Work out the finished part from the listing and answer in its coordinate system (mm). A direction names the side the tool comes from. Give positions to 0.01 mm unless a question says otherwise; leave off trailing zeros. Loops run counter-clockwise (first coordinate to the right, second up) from the corner with the lowest first, then second, coordinate; pieces in that order, holes last. Notation, with made-up numbers: (-15.5, 53) - (10.5, 53) arc R24 cw to (10.5, 68) - close; hole circle Ø3 at (-37, 37.5). An arc over 180 degrees is marked (long way). Use CSV: the item, a comma, the result in double quotes.
from build123d import *

# Parameters (mm, degrees)
SKETCH1_W           = 175
SKETCH1_H           = 43
BOSS_EXTRUDE1_DEPTH = 4
BOSS_EXTRUDE2_DEPTH = 43
SKETCH2_R           = 1.55
SKETCH2_W           = 24.921803412
SKETCH2_H           = 2.5
CUT_EXTRUDE1_DEPTH  = 43
SKETCH3_R           = 1.6
SKETCH3_R_2         = 8
SKETCH3_R_3         = 4.1
CUT_EXTRUDE2_DEPTH  = 43
SKETCH4_R           = 5
CUT_EXTRUDE3_DEPTH  = 43
CUT_EXTRUDE4_DEPTH  = 5
SKETCH6_W           = 101
SKETCH6_H           = 32.974785191
BOSS_EXTRUDE3_DEPTH = 3
CUT_EXTRUDE6_DEPTH  = 1.25
CUT_EXTRUDE7_DEPTH  = 3
CUT_EXTRUDE8_DEPTH  = 4
SKETCH4_4_R         = 4.1
CUT_EXTRUDE9_DEPTH  = 150
BOSS_EXTRUDE4_DEPTH = 60
CUT_EXTRUDE10_DEPTH = 50
BOSS_EXTRUDE5_DEPTH = 1.5
BOSS_EXTRUDE6_DEPTH = 3


with BuildPart() as part:
    # Sketch1 → Boss-Extrude1 (new body)
    with BuildSketch(Plane(origin=(0, 0, 0), x_dir=(1, 0, 0), z_dir=(0, 1, 0))):
        Rectangle(SKETCH1_W, SKETCH1_H)
        Polygon((77.5, -17.02423389), (-18.39852542, -17.02423389), (77.5, 12.216270532), align=None, mode=Mode.SUBTRACT)
        Polygon((-23.5, -13.411203118), (-23.5, 17.839340837), (77.209154002, 17.839340837), align=None, mode=Mode.SUBTRACT)
        Polygon((-33.5, -8.231428571), (-79.616903449, 16.459632181), (-33.5, 16.459632181), align=None, mode=Mode.SUBTRACT)
        Polygon((-80.5, -17.02423389), (-80.5, 9.251394926), (-36.98536512, -17.02423389), align=None, mode=Mode.SUBTRACT)
    extrude(amount=BOSS_EXTRUDE1_DEPTH)

    # Sketch1_3 → Boss-Extrude2 (add)
    with BuildSketch(Plane(origin=(0, 0, 0), x_dir=(1, 0, 0), z_dir=(0, 1, 0))):
        Polygon((-87.5, 21.5), (-87.5, -21.5), (-80.5, -21.5), (-80.5, -17.02423389), (-80.5, 9.251394926), (-80.5, 21.5), align=None)
        Polygon((-33.5, -8.231428571), (-33.5, -21.5), (-23.5, -21.5), (-23.5, -13.411203118), (-23.5, 17.839340837), (-23.5, 21.5), (-33.5, 21.5), (-33.5, 16.459632181), align=None)
        Polygon((77.5, -17.02423389), (77.5, -21.5), (87.5, -21.5), (87.5, 21.5), (77.5, 21.5), (77.5, 12.216270532), align=None)
    extrude(amount=-BOSS_EXTRUDE2_DEPTH)

    # Sketch2 → Cut-Extrude1 (cut)
    with BuildSketch(Plane(origin=(-80.5, 0, 0), x_dir=(0, 0, -1), z_dir=(1, 0, 0))):
        Polygon((21.5, -43), (21.5, -30.260907637), (14.145081595, -43), align=None)
        Polygon((-21.5, -43), (-14.145081595, -43), (-21.5, -30.260907637), align=None)
        with Locations((0, -34)):
            Circle(SKETCH2_R)
        with Locations((-10.825317547, -27.75)):
            Circle(SKETCH2_R)
        with Locations((-10.825317547, -15.25)):
            Circle(SKETCH2_R)
        with Locations((0, 2.75)):
            Rectangle(SKETCH2_W, SKETCH2_H)
        with Locations((0, -9)):
            Circle(SKETCH2_R)
        with Locations((10.825317547, -15.25)):
            Circle(SKETCH2_R)
        with Locations((10.825317547, -27.75)):
            Circle(SKETCH2_R)
    extrude(amount=-CUT_EXTRUDE1_DEPTH, mode=Mode.SUBTRACT)

    # Sketch3 → Cut-Extrude2 (cut)
    with BuildSketch(Plane(origin=(-23.5, 0, 0), x_dir=(0, 0, -1), z_dir=(1, 0, 0))):
        with Locations((15.5, -37)):
            Circle(SKETCH3_R)
        with Locations((0, -21.5)):
            Circle(SKETCH3_R_2)
        with BuildLine():
            Line((-8, -43), (8, -43))
            Line((8, -43), (8, -21.5))
            ThreePointArc((8, -21.5), (0, -29.5), (-8, -21.5))
            Line((-8, -21.5), (-8, -43))
        make_face()
        with Locations((18.5, -21.5)):
            Circle(SKETCH3_R_3)
        with Locations((15.5, -6)):
            Circle(SKETCH3_R)
        with Locations((-15.5, -6)):
            Circle(SKETCH3_R)
        with Locations((-18.5, -21.5)):
            Circle(SKETCH3_R_3)
        with Locations((-15.5, -37)):
            Circle(SKETCH3_R)
    extrude(amount=-CUT_EXTRUDE2_DEPTH, mode=Mode.SUBTRACT)

    # Sketch4 → Cut-Extrude3 (cut)
    with BuildSketch(Plane(origin=(87.5, 0, 0), x_dir=(0, 0, -1), z_dir=(1, 0, 0))):
        with Locations((0, -21.5)):
            Circle(SKETCH4_R)
        with BuildLine():
            ThreePointArc((21.5, -18.705362278), (16.998334258, -17.684898429), (14.4, -21.5))
            ThreePointArc((14.4, -21.5), (16.998334258, -25.315101571), (21.5, -24.294637722))
            Line((21.5, -24.294637722), (21.5, -18.705362278))
        make_face()
        with BuildLine():
            ThreePointArc((-21.5, -24.294637722), (-16.998334258, -25.315101571), (-14.4, -21.5))
            ThreePointArc((-14.4, -21.5), (-16.998334258, -17.684898429), (-21.5, -18.705362278))
            Line((-21.5, -18.705362278), (-21.5, -24.294637722))
        make_face()
        with BuildLine():
            Line((-6, -43), (6, -43))
            Line((6, -43), (6, -37.5))
            ThreePointArc((6, -37.5), (0, -31.5), (-6, -37.5))
            Line((-6, -37.5), (-6, -43))
        make_face()
    extrude(amount=-CUT_EXTRUDE3_DEPTH, mode=Mode.SUBTRACT)

    # Sketch4_3 → Cut-Extrude4 (cut)
    with BuildSketch(Plane(origin=(87.5, 0, 0), x_dir=(0, 0, -1), z_dir=(1, 0, 0))):
        with BuildLine():
            ThreePointArc((-8.05, -21.5), (0, -29.55), (8.05, -21.5))
            Line((8.05, -21.5), (5, -21.5))
            ThreePointArc((5, -21.5), (0, -26.5), (-5, -21.5))
            Line((-5, -21.5), (-8.05, -21.5))
        make_face()
        with BuildLine():
            Line((5, -21.5), (8.05, -21.5))
            ThreePointArc((8.05, -21.5), (0, -13.45), (-8.05, -21.5))
            Line((-8.05, -21.5), (-5, -21.5))
            ThreePointArc((-5, -21.5), (0, -16.5), (5, -21.5))
        make_face()
    extrude(amount=-CUT_EXTRUDE4_DEPTH, mode=Mode.SUBTRACT)

    # Sketch6 → Boss-Extrude3 (add)
    with BuildSketch(Plane(origin=(0, 0, -21.5), x_dir=(-1, 0, 0), z_dir=(0, 0, -1))):
        Polygon((87.5, -30.260907637), (80.5, -30.260907637), (33.5, -43), (23.5, -43), (-77.5, -43), (-87.5, -43), (-87.5, 4), (87.5, 4), align=None)
        with Locations((-27, -18.169210683)):
            Rectangle(SKETCH6_W, SKETCH6_H, mode=Mode.SUBTRACT)
        Polygon((80.5, -23.601473433), (80.5, -1.681818087), (33.5, -1.681818087), (33.5, -34.656603278), align=None, mode=Mode.SUBTRACT)
    boss_extrude3 = extrude(amount=BOSS_EXTRUDE3_DEPTH)

    # Mirror1: Boss-Extrude3 across plane
    add(boss_extrude3.mirror(Plane.XY))

    # Sketch7 → Cut-Extrude6 (cut, symmetric)
    with BuildSketch(Plane(origin=(81.5, 0, 0), x_dir=(0, 0, -1), z_dir=(1, 0, 0))):
        with BuildLine():
            Line((11.709666808, -33.5), (1.443160895, -31.162233309))
            ThreePointArc((1.443160895, -31.162233309), (0, -31), (-1.443160895, -31.162233309))
            Line((-1.443160895, -31.162233309), (-11.709666808, -33.5))
            ThreePointArc((-11.709666808, -33.5), (-12.278204733, -33.856933451), (-12.5, -34.490529316))
            Line((-12.5, -34.490529316), (-12.5, -59.657999149))
            Line((-12.5, -59.657999149), (12.5, -59.657999149))
            Line((12.5, -59.657999149), (12.5, -34.490529316))
            ThreePointArc((12.5, -34.490529316), (12.278204733, -33.856933451), (11.709666808, -33.5))
        make_face()
    extrude(amount=CUT_EXTRUDE6_DEPTH, both=True, mode=Mode.SUBTRACT)

    # Sketch8 → Cut-Extrude7 (cut)
    with BuildSketch(Plane.ZY.offset(33.5)):
        with BuildLine():
            Line((-8, -43), (-8, -21.5))
            ThreePointArc((-8, -21.5), (0, -13.5), (8, -21.5))
            Line((8, -21.5), (8, -43))
            Line((8, -43), (11.5, -43))
            Line((11.5, -43), (11.5, -21.5))
            ThreePointArc((11.5, -21.5), (0, -10), (-11.5, -21.5))
            Line((-11.5, -21.5), (-11.5, -43))
            Line((-11.5, -43), (-8, -43))
        make_face()
    extrude(amount=-CUT_EXTRUDE7_DEPTH, mode=Mode.SUBTRACT)

    # Sketch9 → Cut-Extrude8 (cut)
    with BuildSketch(Plane(origin=(-80.5, 0, 0), x_dir=(0, 0, -1), z_dir=(1, 0, 0))):
        Polygon((-2.9, -32.325684219), (-2.9, -35.674315781), (0, -37.348631561), (2.9, -35.674315781), (2.9, -32.325684219), (0, -30.651368439), align=None)
        Polygon((-10.825317547, -24.401368439), (-13.725317547, -26.075684219), (-13.725317547, -29.424315781), (-10.825317547, -31.098631561), (-7.925317547, -29.424315781), (-7.925317547, -26.075684219), align=None)
        Polygon((-10.825317547, -18.598631561), (-7.925317547, -16.924315781), (-7.925317547, -13.575684219), (-10.825317547, -11.901368439), (-13.725317547, -13.575684219), (-13.725317547, -16.924315781), align=None)
        Polygon((-2.9, -7.325684219), (-2.9, -10.674315781), (0, -12.348631561), (2.9, -10.674315781), (2.9, -7.325684219), (0, -5.651368439), align=None)
        Polygon((7.925317547, -13.575684219), (7.925317547, -16.924315781), (10.825317547, -18.598631561), (13.725317547, -16.924315781), (13.725317547, -13.575684219), (10.825317547, -11.901368439), align=None)
        Polygon((7.925317547, -26.075684219), (7.925317547, -29.424315781), (10.825317547, -31.098631561), (13.725317547, -29.424315781), (13.725317547, -26.075684219), (10.825317547, -24.401368439), align=None)
    extrude(amount=-CUT_EXTRUDE8_DEPTH, mode=Mode.SUBTRACT)

    # Sketch4_4 → Cut-Extrude9 (cut)
    with BuildSketch(Plane(origin=(87.5, 0, 0), x_dir=(0, 0, -1), z_dir=(1, 0, 0))):
        with Locations((18.5, -21.5)):
            Circle(SKETCH4_4_R)
        with Locations((-18.5, -21.5)):
            Circle(SKETCH4_4_R)
    extrude(amount=-CUT_EXTRUDE9_DEPTH, mode=Mode.SUBTRACT)

    # Sketch10 → Boss-Extrude4 (add)
    with BuildSketch(Plane(origin=(87.5, 0, 0), x_dir=(0, 0, -1), z_dir=(1, 0, 0))):
        with BuildLine():
            Line((7.4, -37.5), (5.4, -37.5))
            ThreePointArc((5.4, -37.5), (0, -32.1), (-5.4, -37.5))
            Line((-5.4, -37.5), (-7.4, -37.5))
            ThreePointArc((-7.4, -37.5), (0, -30.1), (7.4, -37.5))
        make_face()
    extrude(amount=BOSS_EXTRUDE4_DEPTH)

    # Sketch10_2 → Cut-Extrude10 (cut)
    with BuildSketch(Plane(origin=(87.5, 0, 0), x_dir=(0, 0, -1), z_dir=(1, 0, 0))):
        with BuildLine():
            Line((7.4, -37.5), (5.4, -37.5))
            ThreePointArc((5.4, -37.5), (0, -32.1), (-5.4, -37.5))
            Line((-5.4, -37.5), (-7.4, -37.5))
            ThreePointArc((-7.4, -37.5), (0, -30.1), (7.4, -37.5))
        make_face()
    extrude(amount=CUT_EXTRUDE10_DEPTH, mode=Mode.SUBTRACT)


with BuildPart() as cut_extrude10_piece_1:
    # of the separate pieces the step leaves, piece 1, a body of its own (cut_extrude10_pieces)
    add(part.part.solids().sort_by_distance((87.5, 4, -24.5))[0])



with BuildPart() as cut_extrude10_piece_2:
    # of the separate pieces the step leaves, piece 2, a body of its own (cut_extrude10_pieces)
    add(part.part.solids().sort_by_distance((137.5, -37.5, 5.4))[0])


with BuildPart() as cut_extrude10_piece_1_1:
    add(cut_extrude10_piece_1.part)

    add(cut_extrude10_piece_2.part)  # Boss-Extrude5 merges Cut-Extrude10 piece 2
    # Sketch12 → Boss-Extrude5 (add, symmetric)
    with BuildSketch(Plane.XY):
        Polygon((145.706039934, -30.1), (139.486039904, -30.1), (87.5, -1.477036856), (87.5, 1.947629303), align=None)
        Polygon((139.486039904, -31.1), (145.808486256, -31.1), (145.706039934, -30.1), (139.486039904, -30.1), align=None)
    extrude(amount=BOSS_EXTRUDE5_DEPTH, both=True)

    # Sketch13 → Boss-Extrude6 (add)
    with BuildSketch(Plane.XZ.offset(37.5)):
        Polygon((87.5, -16.981213653), (87.5, -14.94799315), (139.669059549, -5.4), (147.5, -6), align=None)
    boss_extrude6 = extrude(amount=-BOSS_EXTRUDE6_DEPTH)

    # Mirror2: Boss-Extrude6 across plane
    add(boss_extrude6.mirror(Plane.XY))


solid = cut_extrude10_piece_1_1.part
Item 1: Given P1, Ø2.5, axis at x = -65.5, z = 23.5, coming from the -Y side; P2, Ø6.5, axis at y = -34.5, z = -1, coming from the +X side; P3, Ø12, axis at x = 47, z = 5.5, coming from the -Y side; P4, Ø9, axis at x = 108.5, z = -9, coming from the +Y side, each flat-ended and moving along its own axis, determine where each tip first touches the part or whether it passes through.
Determined:
P1,"stops at y = -34.67"
P2,"stops at x = 147.5"
P3,"passes through"
P4,"stops at y = -34.5"
Item 2: For faces 1 (the flat face through (-84.5, -29, 12)), 2 (the cylindrical face through (-32, -10, 0)), 3 (the cylindrical face through (142.4, -32.1, -0.1)), determine the directions among +Z, -Z, +X, -X, +Y, -Y from which every point of the face is accessible in a straight line to the end or side of a thin tool.
Determined:
face 1,"none"
face 2,"-Y"
face 3,"+X, -Y"
Item 3: Find the intervals of material crossed by line 1 (X direction, y = -27, z = 17.5); line 2 (Z direction, x = 80, y = -21); line 3 (X direction, y = -12.5, z = -4.5), in increasing order.
Determined:
line 1,"x = -87.5 to -80.5, -33.5 to -23.5, 77.5 to 87.5"
line 2,"z = -24.5 to -22.57, -14.43 to -4.97, 4.97 to 14.43, 22.57 to 24.5"
line 3,"x = -87.5 to -80.5, -30.5 to -23.5, 77.5 to 87.5"
Item 4: A cutting plane is placed at A-A on x = 89.5. Determine the outline of the cut face in (y, z), and give its area (3 significant figures).
Determined:
outline,"(-37.5, -16.62) - (-34.5, -16.62) - (-34.5, -14.58) - (-37.5, -14.58) - close; (-37.5, 14.58) - (-34.5, 14.58) - (-34.5, 16.62) - (-37.5, 16.62) - close; (-2.58, -1.5) - (0.85, -1.5) - (0.85, 1.5) - (-2.58, 1.5) - close"
area,"22.5 mm²"
Item 5: The mould has two halves that part along Y. Classify faces 4 (the flat face through (112.15, -36.021, 10.437)), 5 (the cylindrical face through (-28.43, -17.77, 20.2)), 6 (the flat face through (-83.95, -36.72, 17.77)): pulls with the +Y half, pulls with the -Y half, needs draft (parallel to the pull), parting line crosses it, or undercut.
Determined:
face 4,"needs draft"
face 5,"undercut"
face 6,"pulls with the -Y half"
